Design review of the part built by this model. Coordinates are the model's own, in mm. A direction names the side the tool comes from. Coordinates: 2 decimals unless noted, no trailing zeros. Write each loop counter-clockwise with the first axis right and the second up, starting at its lowest first coordinate (ties: lowest second). Pieces come first, ordered by that corner, then holes. Notation, with made-up numbers: (27, 67) -> (82, 67) arc R8 ccw to (82, 79) -> close; hole circle Ø4 at (23.5, 85.25). An arc over 180 degrees is marked (long way). Write item = value, one per line. Start each with the question number.
```python
from build123d import *

# Parameters (mm, degrees)
F0_W     = 40.2857027948
F0_H     = 12.7
F0_R     = 3.175
F1_DEPTH = 1.5875
F0_W_2   = 1.5875
F2_DEPTH = 7.62
F4_R     = 3.175
F5_DEPTH = 25.4


# Not quite as in the source:
# - a length typed as a fraction of an inch, garbled in the dataset ("3 / 203.2 mm" for 3/8 in), is restored


with BuildPart() as f1:
    # F0 (on Front) → F1 (new body)
    with BuildSketch(Plane.XZ):
        with Locations((-20.1428513974, 0)):
            Rectangle(F0_W, F0_H)
        with Locations((-33.6422286928, 0)):
            Circle(F0_R, mode=Mode.SUBTRACT)
    extrude(amount=F1_DEPTH)

    # F0 (on Front) → F2 (join)
    with BuildSketch(Plane.XZ):
        with Locations((0.79375, 0)):
            Rectangle(F0_W_2, F0_H)
    extrude(amount=F2_DEPTH)

    # F3: F1 across face


with BuildPart() as f1_1:
    add(f1.part)
    add(f1.part.mirror(Plane(origin=(0.79375, -7.62, 0), x_dir=(1, 0, 0), z_dir=(0, -1, 0))))

    # F4 (on face) → F5 (cut)
    with BuildSketch(Plane(origin=(0, 0, 0), x_dir=(0, -1, 0), z_dir=(-1, 0, 0))):
        with Locations((7.62, 0)):
            Circle(F4_R)
    extrude(amount=-F5_DEPTH, mode=Mode.SUBTRACT)


solid = f1_1.part
```
(1) For line 1 (Z direction, x = 0.6, y = -7.62) (3 decimals); line 2 (Y direction, x = -21, z = 4.5); line 3 (X direction, y = -11.5, z = 4.5), list the stretches that pass through material, from the lowest coordinate up.
(2) For faces 4 (the face through (-20, 0, 0)), 5 (the face through (0, -10, -3)), list the 3-axis set-ups (+Z, -Z, +X, -X, +Y, -Y) from which the entire face can be reached by the end or side of a thin tool; tool diameter is ignored.
(3) For pin 1 Ø6 at (y, z) = (-10, 4) entering from -X, flat-tipped, find the tip position at first contact; note if it passes through.
(4) Take a section at A-A, the plane x = -24. State the section outline as (y, z) points, then the cut area to 3 significant figures.
(5) Mouldability with a two-part tool opening along Z and no side actions: class faces 1 (the face through (-40.286, -14, 0)), 2 (the face through (-36.814, -0.783, 0.14)), 3 (the face through (-16, -1, 6.35)) as pulls with the +Z half, pulls with the -Z half, needs draft (parallel to the pull), parting line crosses it, or undercut.
(6) Take a section at C-C, the plane z = 0. State the section outline as (x, y) points (1 decimal).
Report:
q1.line_1 = -6.35 to -3.175, 3.175 to 6.35
q1.line_2 = -15.24 to -13.65, -1.59 to 0
q1.line_3 = 0 to 1.59
q2.face_4 = +Z, -Z, +X, -X, +Y
q2.face_5 = +Z, -Z, -X
q3.pin_1 = 0
q4.outline = (-15.24, -6.35) -> (-13.65, -6.35) -> (-13.65, 6.35) -> (-15.24, 6.35) -> close; (-1.59, -6.35) -> (0, -6.35) -> (0, 6.35) -> (-1.59, 6.35) -> close
q4.area = 40.3 mm2
q5.face_1 = needs draft
q5.face_2 = undercut
q5.face_3 = pulls with the +Z half
q6.outline = (-40.3, -15.2) -> (-36.8, -15.2) -> (-36.8, -13.7) -> (-40.3, -13.7) -> close; (-40.3, -1.6) -> (-36.8, -1.6) -> (-36.8, 0) -> (-40.3, 0) -> close; (-30.5, -15.2) -> (1.6, -15.2) -> (1.6, -10.8) -> (0, -10.8) -> (0, -13.7) -> (-30.5, -13.7) -> close; (-30.5, -1.6) -> (0, -1.6) -> (0, -4.4) -> (1.6, -4.4) -> (1.6, 0) -> (-30.5, 0) -> close
